Check sheet for the drawn part. Datum: minimum x, y, z corner. Units: mm. Coordinates: 2 decimals unless noted, no trailing zeros. Write each loop counter-clockwise with the first axis right and the second up, starting at its lowest first coordinate (ties: lowest second). Pieces come first, ordered by that corner, then holes. Notation, with made-up numbers: (50.5, 33.5) - (106.5, 33.5) arc R31 cw to (106.5, 61.5) - close; hole circle Ø8 at (21, 37). An arc over 180 degrees is marked (long way). Write each question's results on one line, items separated by ' | '.
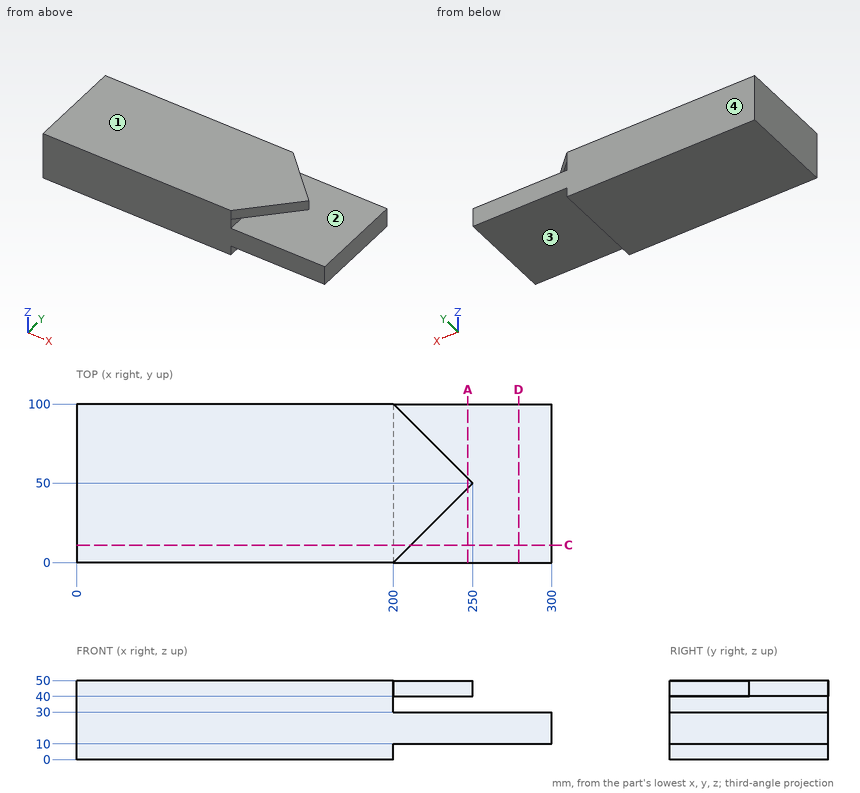
1. Sectioned sample at C-C (y = 11). Record the cut outline in (x, z), then the cut area to 3 significant figures.
Values follow:
outline: (0, 0) - (200, 0) - (200, 10) - (300, 10) - (300, 30) - (200, 30) - (200, 40) - (211, 40) - (211, 50) - (0, 50) - close | area: 12,100 mm^2
2. Sectioned sample at A-A (x = 247). Record the cut outline in (y, z).
Values follow:
outline: (0, 10) - (100, 10) - (100, 30) - (0, 30) - close; (47, 40) - (53, 40) - (53, 50) - (47, 50) - close
3. Go/stop test with flat-tipped pins: pin 1 (2 mm diameter, centred on x = 83.5, y = 58.5, fed in from -Z); pin 2 (5 mm diameter, centred on y = 64, z = 33, fed in from +X); pin 3 (15 mm diameter, centred on x = 217, y = 53.5, fed in from -Z). Record where each tip stops, or that it passes through.
Values follow:
pin 1: stops at z = 0 | pin 2: stops at x = 200 | pin 3: stops at z = 10
4. Material ranges on L1, parallel to Z at x = 268, y = 63; L2, parallel to X at y = 19, z = 7; L3, parallel to Y at x = 210, z = 41.5, recorded low to high. Write a range as [from, to].
Values follow:
L1: z = [10, 30] | L2: x = [0, 200] | L3: y = [10, 90]
5. Sectioned sample at D-D (x = 279). Record the cut outline in (y, z).
Values follow:
outline: (0, 10) - (100, 10) - (100, 30) - (0, 30) - close
6. Draft check along Z on the marked faces 1, 2, 3 and 4. Enter one of: pulls with the +Z half, pulls with the -Z half, needs draft (parallel to the pull), parting line crosses it, or undercut.
Values follow:
face 1: pulls with the +Z half | face 2: undercut | face 3: pulls with the -Z half | face 4: needs draft
